Read the model definition and answer for the solid it produces. Units are mm, in the model's axes. Round coordinates to 2 decimals unless told otherwise and drop trailing zeros. Order: outer loops, then holes, each group sorted by start corner. A loop starts at its lowest first (then second) coordinate and runs counter-clockwise, first axis right, second up. Notation, with made-up numbers: (46.5, -16) -> (89.5, -16) arc R18 ccw to (89.5, 4) -> close; hole circle Ø10 at (54.5, 85). An arc over 180 degrees is marked (long way). Use a Markdown table: item, result. Add a question column.
1. Consider L1, parallel to Y at x = -5.5, z = 6; L2, parallel to Y at x = 23, z = 5.5; L3, parallel to X at y = -26.5, z = 4.5 (3 decimals). Determine where each line is inside the solid, lowest interval first. Write a range as [from, to].
2. Section C-C, the plane z = 2.25 is taken. Give the vertices of the cut face in (x, y), then the cut area to 3 significant figures.
3. Given pin 1 (3 mm diameter, centred on x = 4.5, y = -28.5, fed in from +Z); pin 2 (1.5 mm diameter, centred on y = 2.5, z = 1.5, fed in from -X), each flat-ended and moving along its own axis, determine where each tip first touches the part or whether it passes through.
```python
from build123d import *

# Parameters (mm, degrees)
F0_R     = 11
F1_DEPTH = 7
F2_SIZE  = 3.49999


# Not quite as in the source:
# - a fillet or chamfer is up to 0.001 mm smaller than in the source, because OpenCascade refuses the exact size


with BuildPart() as f1:
    # F0 (on Top) → F1 (new body)
    with BuildSketch(Plane.XY):
        Polygon((28.3908957982, 27.4554844946), (0, 91.3447894481), (-28.3908957982, 27.4554844946), (-18.890943275, 10.8594947502), (-37.9725949446, 10.8594947502), (-79.1069081654, -45.6723947241), (-9.5816991464, -38.3149792447), (0.0408733116, -21.7897841527), (9.5816991464, -38.3149792447), (79.1069081654, -45.6723947241), (37.9725949446, 10.8594947502), (18.8500699634, 10.9302894025), align=None)
        with Locations((-31.8169734902, -18.3695382094)):
            Circle(F0_R, mode=Mode.SUBTRACT)
        with Locations((31.8169734902, -18.3695382094)):
            Circle(F0_R, mode=Mode.SUBTRACT)
        Circle(F0_R, mode=Mode.SUBTRACT)
        with Locations((0, 36.7390764187)):
            Circle(F0_R, mode=Mode.SUBTRACT)
    extrude(amount=F1_DEPTH)

    # F2 (size 3.5 in the source; OpenCascade refuses exactly that, so slightly less here)
    f2_edges = [f1.edges().sort_by_distance(p)[0] for p in [
        (-44.344304, -41.993687, 7),
        (-4.770413, -30.052382, 0),
        (-44.344304, -41.993687, 0),
        (-4.770413, -30.052382, 7),
        (4.811286, -30.052382, 7),
        (4.811286, -30.052382, 0),
        (44.344304, -41.993687, 7),
        (44.344304, -41.993687, 0),
        (-58.539752, -17.40645, 7),
        (58.539752, -17.40645, 7),
        (-14.195448, 59.400137, 7),
        (14.195448, 59.400137, 7),
        (-28.431769, 10.859495, 7),
        (-23.64092, 19.15749, 7),
        (23.620483, 19.192887, 0),
        (28.411332, 10.894892, 7),
        (23.620483, 19.192887, 7),
        (-28.431769, 10.859495, 0),
        (-58.539752, -17.40645, 0),
        (-14.195448, 59.400137, 0),
        (14.195448, 59.400137, 0),
        (58.539752, -17.40645, 0),
        (28.411332, 10.894892, 0),
    ]]
    chamfer(f2_edges, length=F2_SIZE)


solid = f1.part
```
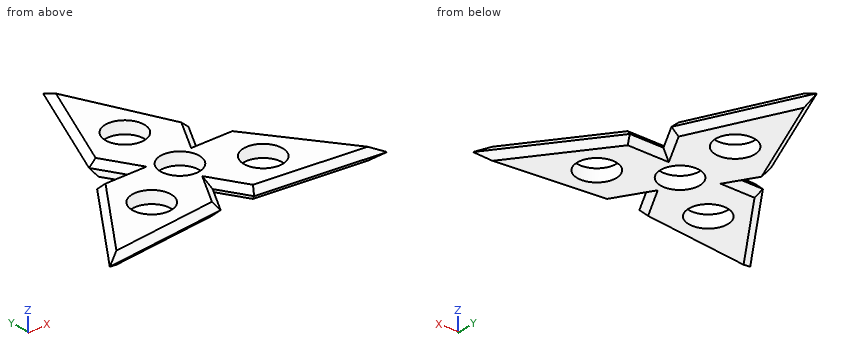
Verdict:
| question | item | result |
|---|---|---|
| 1 | L1 | y = [-26.34, -9.53], [9.53, 27.21], [46.27, 72.81] |
| 1 | L2 | y = [-37.72, -24.95], [-11.79, 8.91], [22.12, 34.66] |
| 1 | L3 | x = [-63.92, -39.226], [-24.408, -3.859], [3.915, 24.408], [39.226, 63.92] |
| 2 | outline | (-76.44, -44.13) -> (-10.34, -37.14) -> (0.05, -19.3) -> (10.35, -37.14) -> (76.44, -44.13) -> (37.33, 9.61) -> (16.69, 9.69) -> (26.99, 27.53) -> (0, 88.27) -> (-27.62, 26.11) -> (-18.18, 9.61) -> (-37.34, 9.61) -> close; hole circle Ø22 at (-31.82, -18.37); hole circle Ø22 at (0, 0); hole circle Ø22 at (0, 36.74); hole circle Ø22 at (31.82, -18.37) |
| 2 | area | 6,250 mm2 |
| 3 | pin 1 | stops at z = 5.51 |
| 3 | pin 2 | stops at x = -42.66 |
